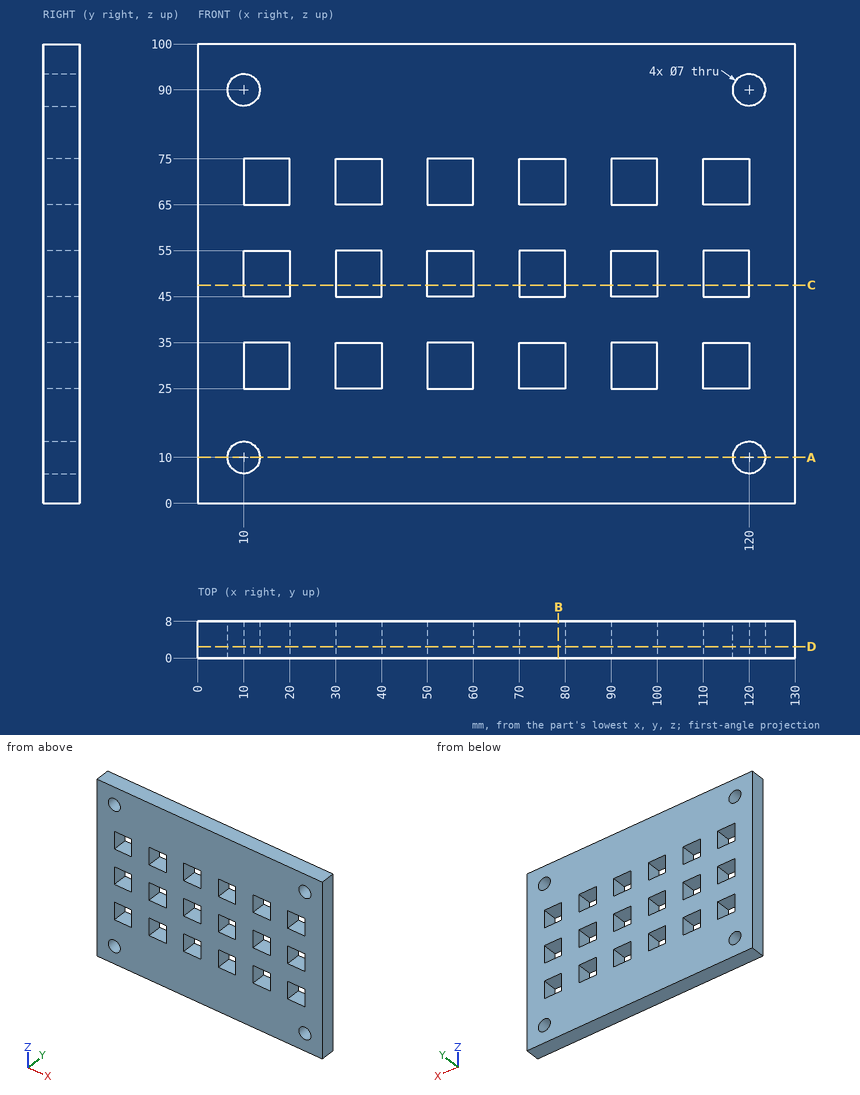
Could you check a few things on this drawing? It's one solid part, dimensions in mm from its lowest x, y, z. Give positions to 0.01 mm unless a question says otherwise; leave off trailing zeros. Order: outer loops, then holes, each group sorted by start corner. A loop starts at its lowest first (then second) coordinate and runs counter-clockwise, first axis right, second up. Notation, with made-up numbers: M 63.5,2.5 L 79.5,2.5 A18 cw 79.5,10.5 Z; hole C 41.5,35.25 d3. An arc over 180 degrees is marked long. Use one line per item in the form item = value. Start each with the question number.
Item 1: If we section it at A-A (z = 10): Write out the boundary of the cut face in (x, y), then the cut area to 3 significant figures.
Item 2: If we section it at C-C (z = 47.5): Write out the boundary of the cut face in (x, y), then the cut area to 3 significant figures.
Item 3: If we section it at D-D (y = 2.5): State how many separate pieces and enclosed holes the cut face has, then the cut area to 3 significant figures.
Item 4: If we section it at B-B (x = 78.5): Write out the boundary of the cut face in (y, z).
Item 5: If I drill on line 1 along Z through (x, y) = (17, 2.25); line 2 along X through (y, z) = (4, 10); line 3 along Z through (x, y) = (7, 5.5), over which ranges is the centre line in solid material (lowest first)?
Outcome:
q1.outline = M 0,0 L 6.5,0 L 6.5,8 L 0,8 Z; M 13.5,0 L 116.5,0 L 116.5,8 L 13.5,8 Z; M 123.5,0 L 130,0 L 130,8 L 123.5,8 Z
q1.area = 928 mm2
q2.outline = M 0,0 L 10,0 L 10,8 L 0,8 Z; M 20,0 L 30,0 L 30,8 L 20,8 Z; M 40,0 L 50,0 L 50,8 L 40,8 Z; M 60,0 L 70,0 L 70,8 L 60,8 Z; M 80,0 L 90,0 L 90,8 L 80,8 Z; M 100,0 L 110,0 L 110,8 L 100,8 Z; M 120,0 L 130,0 L 130,8 L 120,8 Z
q2.area = 560 mm2
q3.separate_pieces = 1
q3.enclosed_holes = 22
q3.area = 11,000 mm2
q4.outline = M 0,0 L 8,0 L 8,25 L 0,25 Z; M 0,35 L 8,35 L 8,45 L 0,45 Z; M 0,55 L 8,55 L 8,65 L 0,65 Z; M 0,75 L 8,75 L 8,100 L 0,100 Z
q5.line_1 = 0 to 25, 35 to 45, 55 to 65, 75 to 100
q5.line_2 = 0 to 6.5, 13.5 to 116.5, 123.5 to 130
q5.line_3 = 0 to 8.2, 11.8 to 88.2, 91.8 to 100
